Design review of the part built by this model. Coordinates are the model's own, in mm. A direction names the side the tool comes from. Give positions to 0.01 mm unless a question says otherwise; leave off trailing zeros. Loops run counter-clockwise (first coordinate to the right, second up) from the corner with the lowest first, then second, coordinate; pieces in that order, holes last. Notation, with made-up numbers: (78, -32) -> (134, -32) arc R17 ccw to (134, -24) -> close; hole circle Ø5 at (-10, 52). An arc over 180 degrees is marked (long way). Use a Markdown table: item, result. Add a question column.
1. For pin 1 Ø5 at (x, y) = (11.5, 1.5) entering from +Z; pin 2 Ø2.5 at (x, y) = (43.5, 4) entering from +Z; pin 3 Ø1.8 at (x, y) = (27, 3.5) entering from -Z, all flat-tipped, find the tip position at first contact; note any pin that passes through.
2. To check wall thickness, follow line 1 (X direction, y = 1.5, z = -17); line 2 (Y direction, x = 28, z = 20); line 3 (Z direction, x = 22, y = 6). State the ranges of each line that lie inside material, in increasing order.
3. Add section B-B (x = 10). State the section outline as (y, z) points, and give its area (3 significant figures).
4. Add section A-A (y = 1.25). State the section outline as (x, z) points, and give its area (3 significant figures).
5. Add section C-C (z = -12.5). State the section outline as (x, y) points, and give its area (3 significant figures).
6. For faces 1 (the flat face through (21, 7.053, 30)), 2 (the flat face through (43.766, 2, 0)), 3 (the flat face through (42.766, 4, 0)), list the 3-axis set-ups (+Z, -Z, +X, -X, +Y, -Y) from which the entire face can be reached by the end or side of a thin tool; tool diameter is ignored.
```python
from build123d import *

# Parameters (mm, degrees)
F1_DEPTH = 25
F2_W     = 40.895786
F2_H     = 2.828645
F3_DEPTH = 1
F5_DEPTH = 40.895786
F6_R     = 1
F7_R     = 2


with BuildPart() as f1:
    # F0 (on Top) → F1 (new body, symmetric)
    with BuildSketch(Plane.XY):
        Polygon((42.765886, 0), (0, 0), (0, -1), (43.765886, -1), (43.765886, 6.060815), (51.214214, 6.117835), (51.206559, 7.117806), (42.765886, 7.053189), align=None)
    extrude(amount=F1_DEPTH, both=True)

    # F2 (on face) → F3 (join, through all)
    with BuildSketch(Plane(origin=(0, 0, 0), x_dir=(-1, 0, 0), z_dir=(0, 1, 0))):
        with Locations((-20.447893, 26.414322)):
            Rectangle(F2_W, F2_H)
    extrude(amount=-F3_DEPTH)

    # F4 (on face) → F5 (join, through all)
    with BuildSketch(Plane.YZ.offset(40.895786)):
        Polygon((7.053189, 27.828645), (0, 27.828645), (0, 26.828645), (8.053189, 26.828645), (8.053189, 31.7876), (7.053189, 31.7876), align=None)
    extrude(amount=-F5_DEPTH)

    # F6
    f6_edges = [f1.edges().sort_by_distance(p)[0] for p in [
        (20.447893, 7.053189, 27.828645),
    ]]
    fillet(f6_edges, radius=F6_R)

    # F7
    f7_edges = [f1.edges().sort_by_distance(p)[0] for p in [
        (20.447893, 8.053189, 26.828645),
    ]]
    fillet(f7_edges, radius=F7_R)


solid = f1.part
```
Taken from the geometry:
| question | item | result |
|---|---|---|
| 1 | pin 1 | stops at z = 27.83 |
| 1 | pin 2 | stops at z = 25 |
| 1 | pin 3 | stops at z = 26.83 |
| 2 | line 1 | x = 42.77 to 43.77 |
| 2 | line 2 | y = -1 to 0 |
| 2 | line 3 | z = 26.83 to 27.83 |
| 3 | outline | (-1, -25) -> (0, -25) -> (0, 26.83) -> (6.05, 26.83) arc R2 ccw to (8.05, 28.83) -> (8.05, 31.79) -> (7.05, 31.79) -> (7.05, 28.83) arc R1 cw to (6.05, 27.83) -> (-1, 27.83) -> close |
| 3 | area | 64.2 mm^2 |
| 4 | outline | (0, 26.83) -> (40.9, 26.83) -> (40.9, 27.83) -> (0, 27.83) -> close; (42.77, -25) -> (43.77, -25) -> (43.77, 25) -> (42.77, 25) -> close |
| 4 | area | 90.9 mm^2 |
| 5 | outline | (0, -1) -> (43.77, -1) -> (43.77, 6.06) -> (51.21, 6.12) -> (51.21, 7.12) -> (42.77, 7.05) -> (42.77, 0) -> (0, 0) -> close |
| 5 | area | 58.3 mm^2 |
| 6 | face 1 | +Z, +X, -X, -Y |
| 6 | face 2 | +Z, -Z, +X, -Y |
| 6 | face 3 | +Z, -Z, -X, +Y |
